Job drawing, mm, ordinate dimensions from the low corner. One solid piece. A direction names the side the tool comes from. Round coordinates to 2 decimals unless told otherwise and drop trailing zeros. Order: outer loops, then holes, each group sorted by start corner. A loop starts at its lowest first (then second) coordinate and runs counter-clockwise, first axis right, second up. Notation, with made-up numbers: (5, -12) -> (20, -12) arc R5 ccw to (20, -8) -> close; hole circle Ø11 at (4.5, 20.25). An arc over 180 degrees is marked (long way). Use CSV: the item, a comma, the result in double quotes.
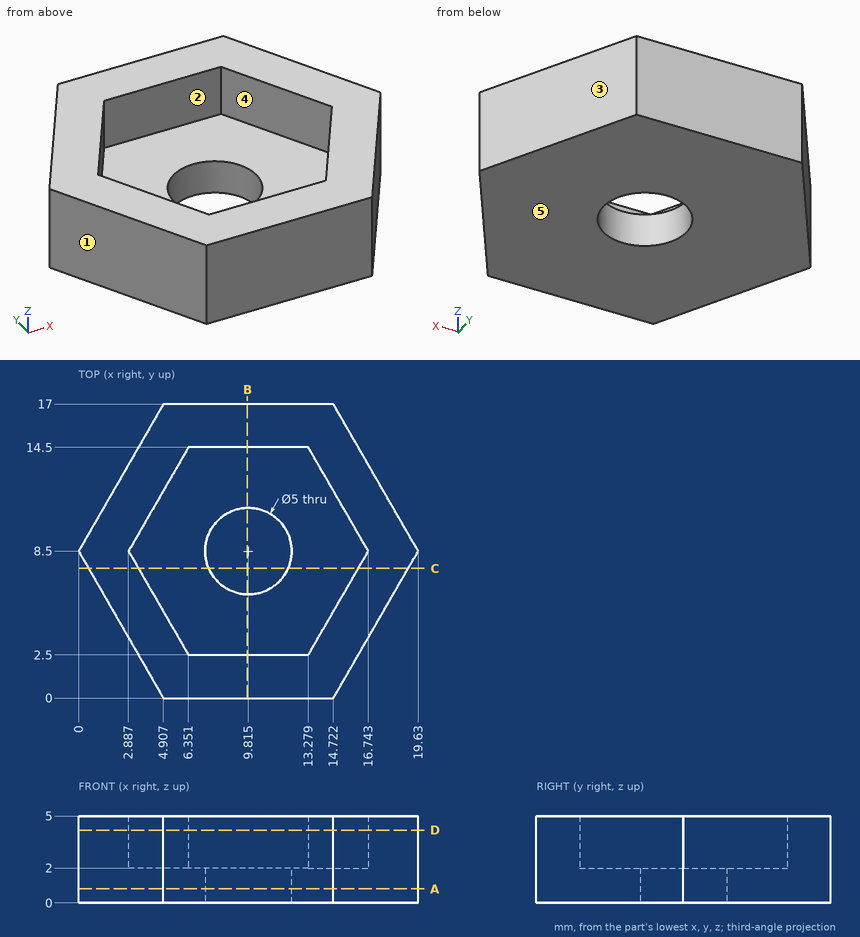
(1) Cut at C-C, the plane y = 7.5. Give the cut face in (x, z) (1 decimal).
Reply:
outline,"(0.6, 0) -> (7.5, 0) -> (7.5, 2) -> (3.5, 2) -> (3.5, 5) -> (0.6, 5) -> close; (12.1, 0) -> (19.1, 0) -> (19.1, 5) -> (16.2, 5) -> (16.2, 2) -> (12.1, 2) -> close"
(2) Cut at B-B, the plane x = 9.75. Give the cut face in (y, z), then the cut area to 3 significant figures.
Reply:
outline,"(0, 0) -> (6, 0) -> (6, 2) -> (2.5, 2) -> (2.5, 5) -> (0, 5) -> close; (11, 0) -> (17, 0) -> (17, 5) -> (14.5, 5) -> (14.5, 2) -> (11, 2) -> close"
area,"39.0 mm2"
(3) Cut at A-A, the plane z = 0.8. Give the cut face in (x, y) (1 decimal).
Reply:
outline,"(0, 8.5) -> (4.9, 0) -> (14.7, 0) -> (19.6, 8.5) -> (14.7, 17) -> (4.9, 17) -> close; hole circle Ø5 at (9.8, 8.5)"
(4) Probe probe 1 along Y at (x, z) = (9.5, 4.1); probe 2 along Z at (x, y) = (14, 10); probe 3 along Y at (x, z) = (15.25, 2.25) (1 decimal). List the from-to ranges inside material, lowest first. Write a range as [from, to].
Reply:
probe 1,"[0, 2.5], [14.5, 17]"
probe 2,"[0, 2]"
probe 3,"[0.9, 5.9], [11.1, 16.1]"
(5) Which spindle directions (+Z, -Z, +X, -X, +Y, -Y) get a long thin tool onto all of the face, cutting with end or side? Do the marked faces 1 and 2. Say none if no direction does.
Reply:
face 1,"+Z, -Z, -X, -Y"
face 2,"+Z"
(6) Pull direction X, two halves, no side cores. Call the marked faces 3, 4 and 5: released by +X, released by -X, zero draft, split by the parting line, or undercut.
Reply:
face 3,"released by +X"
face 4,"undercut"
face 5,"zero draft"
(7) Cut at D-D, the plane z = 4.2. Give the cut face in (x, y).
Reply:
outline,"(0, 8.5) -> (4.91, 0) -> (14.72, 0) -> (19.63, 8.5) -> (14.72, 17) -> (4.91, 17) -> close; hole (2.89, 8.5) -> (6.35, 2.5) -> (13.28, 2.5) -> (16.74, 8.5) -> (13.28, 14.5) -> (6.35, 14.5) -> close"
(8) Drop flat-ended pins along their axis: P1, Ø3, axis at y = 14.5, z = 1.5, coming from the -X side; P2, Ø1.5, axis at y = 2, z = 1.5, coming from the -X side; P3, Ø2, axis at y = 10, z = 0.5, coming from the +X side. Give the stop position or say it passes through.
Reply:
P1,"x = 2.6"
P2,"x = 3.32"
P3,"x = 19.34"
